Verification items for the finished model (mm, model axes). A direction names the side the tool comes from. Round coordinates to 2 decimals unless told otherwise and drop trailing zeros. Write each loop counter-clockwise with the first axis right and the second up, starting at its lowest first coordinate (ties: lowest second). Pieces come first, ordered by that corner, then holes. Notation, with made-up numbers: M 76,-32 L 131,-32 A28 cw 131,-2 Z; hole C 43,-9 d10. An arc over 180 degrees is marked long. One line per item, written item: value. Start each with the question number.
from build123d import *

# Parameters (mm, degrees)
F2_DEPTH = 4


# Not quite as in the source:
# - the program builds the solid bodies; features that only make, move or delete a surface that nothing else refers to are left out


with BuildPart() as f2:
    # F0 (on Front) → F2 (new body, symmetric)
    with BuildSketch(Plane.XZ):
        Polygon((-12.8808012232, 34.1780185699), (-15.9405209124, 13.6672500521), (-8.9405209124, 13.6672500521), (-6.189699587, 32.1073246897), (0, 36.6672500521), (6.189699587, 32.1073246897), (8.9405209124, 13.6672500521), (15.9405209124, 13.6672500521), (12.8808012232, 34.1780185699), (0, 43.6672500521), align=None)
    extrude(amount=F2_DEPTH, both=True)


solid = f2.part
1) Cross-section at C-C (z = 17.5). Record the boundary of the cut face in (x, y), then the cut area to 3 significant figures.
2) Mould release check, pull along X, two halves, no side actions. Record for faces 1 (the flat face through (-12, 0, 13.667)), 2 (the flat face through (7.546, -0.056, 23.016)), 3 (the flat face through (3.05, -0.06, 34.42)), 4 (the flat face through (-14.39, -0.06, 24.07)): pulls with the +X half, pulls with the -X half, needs draft (parallel to the pull), parting line crosses it, or undercut.
3) Gauge pin test, flat end, axial feed: pin 1 Ø1.5 at (y, z) = (2, 34) entering from +X. Record the tip position at first contact, or that the pin passes through.
4) Cross-section at D-D (x = -11.5). Record the boundary of the cut face in (y, z), then the cut area to 3 significant figures.
5) Cross-section at A-A (z = 33.5). Record the boundary of the cut face in (x, y), then the cut area to 3 significant figures.
6) Cross-section at B-B (y = -3). Record the boundary of the cut face in (x, z).
7) Thickness scan on line 1 (X direction, y = 3.25, z = 24); line 2 (X direction, y = -2.75, z = 36); line 3 (Z direction, x = -9.5, y = -2). Record the ranges inside material, lowest first.
8) Access from +Z, -Z, +X, -X, +Y, -Y to the whole of each face (thin tool, end or side, straight path). Record for faces 5 (the flat face through (6.531, -0.056, 38.856)), 6 (the flat face through (-7.584, -0.056, 22.758)).
Results below:
1. outline: M -15.37,-4 L -8.37,-4 L -8.37,4 L -15.37,4 Z; M 8.37,-4 L 15.37,-4 L 15.37,4 L 8.37,4 Z
1. area: 112 mm²
2. face 1: needs draft
2. face 2: undercut
2. face 3: undercut
2. face 4: pulls with the -X half
3. pin 1: stops at x = 13.02
4. outline: M -4,13.67 L 4,13.67 L 4,35.2 L -4,35.2 Z
4. area: 172 mm²
5. outline: M -12.98,-4 L -4.3,-4 L -4.3,4 L -12.98,4 Z; M 4.3,-4 L 12.98,-4 L 12.98,4 L 4.3,4 Z
5. area: 139 mm²
6. outline: M -15.94,13.67 L -8.94,13.67 L -6.19,32.11 L 0,36.67 L 6.19,32.11 L 8.94,13.67 L 15.94,13.67 L 12.88,34.18 L 0,43.67 L -12.88,34.18 Z
7. line 1: x = -14.4 to -7.4, 7.4 to 14.4
7. line 2: x = -10.41 to -0.91, 0.91 to 10.41
7. line 3: z = 13.67 to 36.67
8. face 5: +Z, +X, +Y, -Y
8. face 6: -Z, +Y, -Y
